Answer from the drawing. Dimensions are ordinates in mm from the lowest x, y and z of the part. A direction names the side the tool comes from. Round coordinates to 2 decimals unless told otherwise and drop trailing zeros. Write each loop counter-clockwise with the first axis right and the second up, starting at its lowest first coordinate (ties: lowest second). Pieces come first, ordered by that corner, then holes. Notation, with made-up numbers: (17, 67.25) - (37, 67.25) arc R33 cw to (37, 99.25) - close; hole circle Ø8 at (75.25, 80.25). An arc over 180 degrees is marked (long way). Answer in a Markdown table with one row per item.
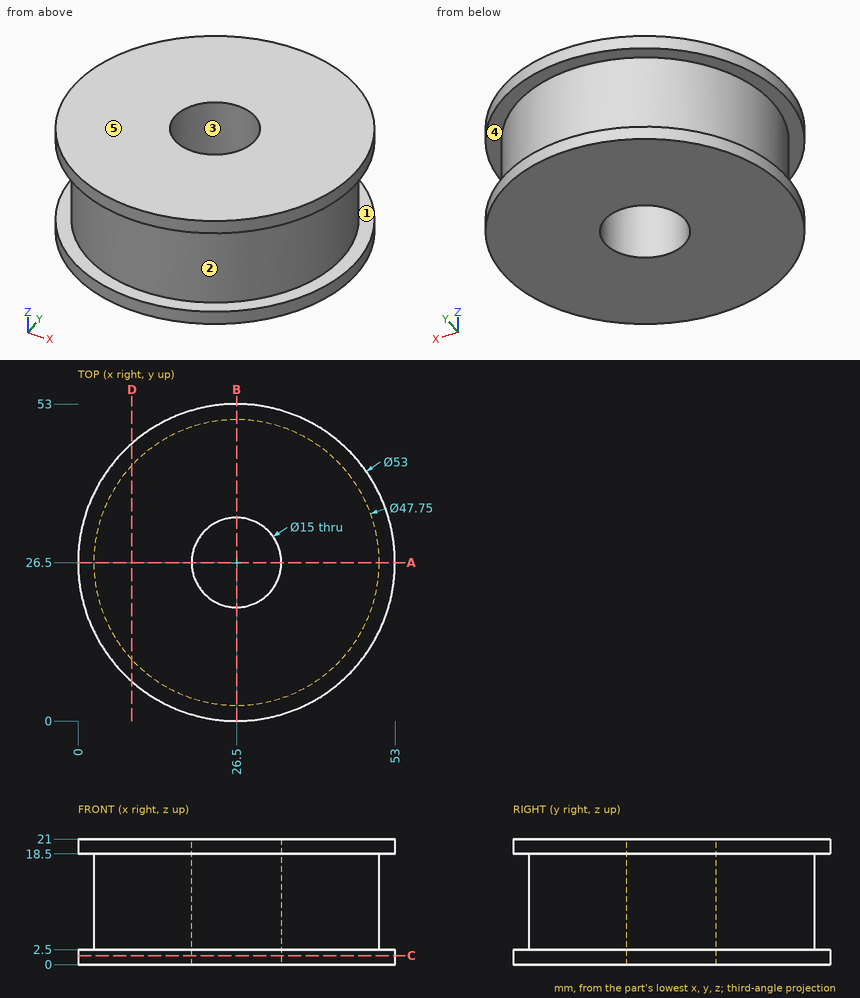
(1) Find the intervals of material crossed by line 1 (Y direction, x = 26.5, z = 7.5) (3 decimals); line 2 (Z direction, x = 49, y = 37); line 3 (X direction, y = 31, z = 17.5), in increasing order.
Checked values:
| item | result |
|---|---|
| line 1 | y = 2.625 to 19, 34 to 50.375 |
| line 2 | z = 0 to 2.5, 18.5 to 21 |
| line 3 | x = 3.05 to 20.5, 32.5 to 49.95 |
(2) For a pull along X with two mould halves and no side action, classify the marked faces 1, 2 and 3 as pulls with the +X half, pulls with the -X half, needs draft (parallel to the pull), parting line crosses it, or undercut.
Checked values:
| item | result |
|---|---|
| face 1 | needs draft |
| face 2 | parting line crosses it |
| face 3 | undercut |
(3) Section A-A (y = 26.5) is taken. Give the vertices of the cut face in (x, z) (3 decimals).
Checked values:
| item | result |
|---|---|
| outline | (0, 0) - (19, 0) - (19, 21) - (0, 21) - (0, 18.5) - (2.625, 18.5) - (2.625, 2.5) - (0, 2.5) - close; (34, 0) - (53, 0) - (53, 2.5) - (50.375, 2.5) - (50.375, 18.5) - (53, 18.5) - (53, 21) - (34, 21) - close |
(4) Section C-C (z = 1.5) is taken. Give the vertices of the cut face in (x, y), and give its area (3 significant figures).
Checked values:
| item | result |
|---|---|
| outline | circle Ø53 at (26.5, 26.5); hole circle Ø15 at (26.5, 26.5) |
| area | 2,030 mm2 |
(5) Flat-ended cylindrical pins translate along their axes: pin 1 (4 mm diameter, centred on y = 35, z = 8, fed in from +X); pin 2 (5 mm diameter, centred on x = 36.5, z = 18.5, fed in from +Y); pin 3 (4 mm diameter, centred on y = 39, z = 18.5, fed in from +X). Find the tip coordinate at first contact, or state that the pin passes through.
Checked values:
| item | result |
|---|---|
| pin 1 | stops at x = 49.47 |
| pin 2 | stops at y = 51.92 |
| pin 3 | stops at x = 50.83 |
(6) For the marked faces 4 and 5, determine the directions among +Z, -Z, +X, -X, +Y, -Y from which every point of the face is accessible in a straight line to the end or side of a thin tool.
Checked values:
| item | result |
|---|---|
| face 4 | none |
| face 5 | +Z, +X, -X, +Y, -Y |
(7) Section D-D (x = 9) is taken. Give the vertices of the cut face in (y, z), and give its area (3 significant figures).
Checked values:
| item | result |
|---|---|
| outline | (6.6, 0) - (46.4, 0) - (46.4, 2.5) - (42.74, 2.5) - (42.74, 18.5) - (46.4, 18.5) - (46.4, 21) - (6.6, 21) - (6.6, 18.5) - (10.26, 18.5) - (10.26, 2.5) - (6.6, 2.5) - close |
| area | 719 mm2 |
